Source: CAD feature listing. Evaluate the final solid. Frame: model axes, mm. Coordinates: 2 decimals unless noted, no trailing zeros. Order: outer loops, then holes, each group sorted by start corner. A loop starts at its lowest first (then second) coordinate and runs counter-clockwise, first axis right, second up.
Item 1: Ray query, line 1 (Y direction, x = 177, z = 7.5); line 2 (X direction, y = 7.5, z = 10); line 3 (X direction, y = -6.25, z = -2.5). Return the intervals inside material, ascending.
Item 2: Section B-B on x = 0. Return the cut outline in (y, z), then the cut area to 3 significant figures.
Item 3: Contact query for flat-ended pins moving along their axis: P1, Ø9.5, axis at x = -108.5, z = 5.5, coming from the +Y side; P2, Ø5, axis at y = 3.5, z = 3, coming from the +X side. Output: stop coordinate, or through.
Item 4: Section A-A on x = 169.5. Return the cut outline in (y, z).
from build123d import *

# Parameters (mm, degrees)
BOSS_EXTRUDE1_DEPTH   = 4
BOSS_EXTRUDE1_2_DEPTH = 4
SKETCH2_R             = 14
BOSS_EXTRUDE2_DEPTH   = 8.8


with BuildPart() as part:
    # Sketch1 → Boss-Extrude1 (new, symmetric)
    with BuildSketch(Plane(origin=(0, 0, 0), x_dir=(1, 0, 0), z_dir=(0, 1, 0))):
        Polygon((12, -9.7155), (64.77, -17.81175), (183.515, -8.31215), (211.582, -3.0226), (215.9, 0), (211.582, 4.5339), (183.515, 6.80085), (64.77, 14.57325), (12, 9.7155), align=None)
    extrude(amount=BOSS_EXTRUDE1_DEPTH, both=True)



with BuildPart() as body_2:
    # Sketch1 → Boss-Extrude1 2 (new, symmetric)
    with BuildSketch(Plane(origin=(0, 0, 0), x_dir=(1, 0, 0), z_dir=(0, 1, 0))):
        Polygon((-12, -9.7155), (-64.77, -17.81175), (-183.515, -8.31215), (-211.582, -3.0226), (-215.9, 0), (-211.582, 4.5339), (-183.515, 6.80085), (-64.77, 14.57325), (-12, 9.7155), align=None)
    extrude(amount=BOSS_EXTRUDE1_2_DEPTH, both=True)


with BuildPart() as part_1:
    add(part.part)

    add(body_2.part)  # Boss-Extrude2 merges body 2
    # Sketch2 → Boss-Extrude2 (add, symmetric)
    with BuildSketch(Plane(origin=(0, 0, 0), x_dir=(1, 0, 0), z_dir=(0, 1, 0))):
        with Locations(Location((0, 0, 0), (0, 0, 270))):
            Circle(SKETCH2_R)
    extrude(amount=BOSS_EXTRUDE2_DEPTH, both=True)


solid = part_1.part
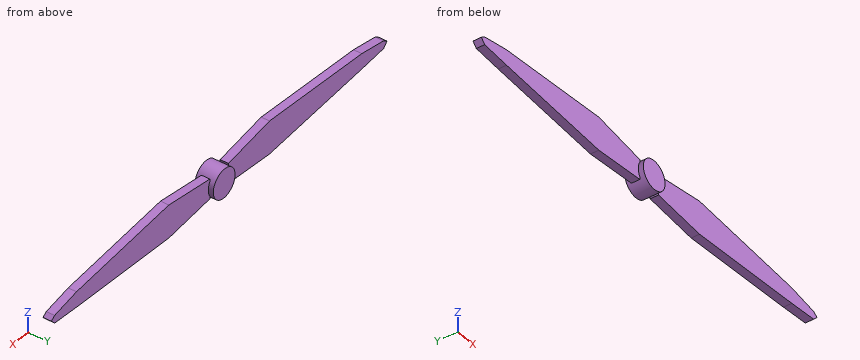
Answer list:
1. line 1: y = -4 to 4
1. line 2: x = -9.8 to 9.8
1. line 3: x = -13.77 to 13.77
2. outline: (-8.8, -14) - (8.8, -14) - (8.8, 14) - (-8.8, 14) - close
2. area: 493 mm2
3. P1: stops at y = 4
3. P2: stops at x = 215.19
4. outline: (-4, -7.72) - (4, -7.72) - (4, 9.43) - (-4, 9.43) - close
